The model under review builds one solid part; all positions refer to its coordinate system, in mm. A direction names the side the tool comes from. Give positions to 0.01 mm unless a question says otherwise; leave off trailing zeros. Order: outer loops, then holes, each group sorted by start corner. A loop starts at its lowest first (then second) coordinate and runs counter-clockwise, first axis right, second up. Notation, with made-up numbers: (-11, 20) - (4, 20) arc R26 ccw to (4, 56) - close; hole circle Ø1 at (55, 8). An arc over 180 degrees is marked (long way). Use CSV: the item, a comma, the result in double quotes. Start each with the question number.
1. Take a section at B-B, the plane x = 65. State the section outline as (y, z) points.
2. Machinability: for faces 1 (the flat face through (10, 13, -16)), 2 (the flat face through (61, 7, -8.5)), 3 (the flat face through (13, 8, -16)), which of the approach directions +Z, -Z, +X, -X, +Y, -Y give a long, thin tool a straight path to every point of the face, cutting with its end or side? Answer none if there is none.
3. Take a section at C-C, the plane z = -19.5. State the section outline as (x, y) points, then the cut area to 3 significant figures.
4. Draft analysis for pull direction Z (two halves, no side actions). For faces 4 (the cylindrical face through (5.81, 6.55, -15.9)), 5 (the flat face through (35, 1, 0)), 6 (the flat face through (9, 7, -46.5)), state which applies: released by +Z, released by -Z, zero draft, split by the parting line, or undercut.
5. Take a section at A-A, the plane z = -65. State the section outline as (x, y) points, then the cut area to 3 significant figures.
6. Take a section at D-D, the plane y = 6.5. State the section outline as (x, z) points.
7. For pin 1 (1 mm diameter, centred on x = 35.5, z = -20.5, fed in from -Y); pin 2 (5 mm diameter, centred on y = 7.5, z = -17, fed in from +X); pin 3 (12 mm diameter, centred on x = 55.5, z = -31.5, fed in from +Y); pin 4 (3 mm diameter, centred on x = 5.5, y = 8, fed in from +Z), all flat-tipped, find the tip position at first contact; note any pin that passes through.
8. To check wall thickness, follow line 1 (X direction, y = 2.1, z = -65); line 2 (Z direction, x = 4, y = 4.25); line 3 (Z direction, x = 65, y = 1). State the ranges of each line that lie inside material, in increasing order. Write a range as [from, to].
```python
from build123d import *

# Parameters (mm, degrees)
SKETCH1_W           = 70
SKETCH1_H           = 70
SKETCH1_R           = 1.7
PLATE_DEPTH         = 3
SKETCH2_W           = 5
SKETCH2_H           = 15
BOSS_EXTRUDE1_DEPTH = 10
FILLET1_R           = 10


with BuildPart() as part:
    # Sketch1 → Plate (new body)
    with BuildSketch(Plane(origin=(0, 0, 0), x_dir=(1, 0, 0), z_dir=(0, 1, 0))):
        with Locations((35, 35)):
            Rectangle(SKETCH1_W, SKETCH1_H)
        with Locations(Location((65, 65, 0), (0, 0, 270))):
            Circle(SKETCH1_R, mode=Mode.SUBTRACT)
        with Locations(Location((5, 65, 0), (0, 0, 90))):
            Circle(SKETCH1_R, mode=Mode.SUBTRACT)
        with Locations(Location((65, 5, 0), (0, 0, 90))):
            Circle(SKETCH1_R, mode=Mode.SUBTRACT)
        with Locations(Location((5, 5, 0), (0, 0, 270))):
            Circle(SKETCH1_R, mode=Mode.SUBTRACT)
    extrude(amount=PLATE_DEPTH)

    # Sketch2 → Boss-Extrude1 (add)
    with BuildSketch(Plane(origin=(0, 3, 0), x_dir=(1, 0, 0), z_dir=(0, 1, 0))):
        with Locations((10.5, 54)):
            Rectangle(SKETCH2_W, SKETCH2_H)
        with Locations((59.5, 54)):
            Rectangle(SKETCH2_W, SKETCH2_H)
        with Locations((10.5, 16)):
            Rectangle(SKETCH2_W, SKETCH2_H)
        with Locations((59.5, 16)):
            Rectangle(SKETCH2_W, SKETCH2_H)
    extrude(amount=BOSS_EXTRUDE1_DEPTH)

    # Fillet1
    # the kernel refuses this fillet: 10 mm, written as the material it adds along each edge
    with BuildSketch(Plane(origin=(8, 3, -22.005102572), x_dir=(-1, 0, 0), z_dir=(0, 0, -1))) as fillet1_piece_1_section:
        with BuildLine():
            CenterArc((10, 9.797958971), FILLET1_R, 180, 78.463040967)
            Line((0, 9.797958971), (-0.2, 9.797958971))
            Line((-0.2, 9.797958971), (-0.2, 0))
            Line((-0.2, 0), (0, -0.2))
            ThreePointArc((0, -0.2), (4, -0.2), (7.96, -0.195959179))
            Line((7.96, -0.195959179), (8, 0))
        make_face()
    fillet1_piece_1 = extrude(amount=39.494897428, mode=Mode.PRIVATE)
    fillet1_piece_1 = split(fillet1_piece_1, bisect_by=Plane(origin=(6.00439902, 5.286170926, -23.5), z_dir=(0, 0, 1)), keep=Keep.TOP, mode=Mode.PRIVATE)
    add(fillet1_piece_1)
    with BuildSketch(Plane(origin=(8, 3, -46.5), x_dir=(-1, 0, 0), z_dir=(0, 0, -1)), Plane(origin=(62, 3, -61.5), x_dir=(1, 0, 0), z_dir=(0, 0, 1)), Plane(origin=(8, 3, -8.5), x_dir=(-1, 0, 0), z_dir=(0, 0, -1)), Plane(origin=(62, 3, -23.5), x_dir=(1, 0, 0), z_dir=(0, 0, 1))) as fillet1_piece_2:
        with BuildLine():
            CenterArc((10, 9.797958971), FILLET1_R, 180, 78.463040967)
            Line((0, 9.797958971), (-0.2, 9.797958971))
            Line((-0.2, 9.797958971), (-0.2, 0))
            Line((-0.2, 0), (0, -0.2))
            ThreePointArc((0, -0.2), (4, -0.2), (7.96, -0.195959179))
            Line((7.96, -0.195959179), (8, 0))
        make_face()
    extrude(amount=15)
    with BuildSketch(Plane(origin=(62, 3, -61.5), x_dir=(1, 0, 0), z_dir=(0, 0, 1))) as fillet1_piece_3_section:
        with BuildLine():
            CenterArc((10, 9.797958971), FILLET1_R, 180, 78.463040967)
            Line((0, 9.797958971), (-0.2, 9.797958971))
            Line((-0.2, 9.797958971), (-0.2, 0))
            Line((-0.2, 0), (0, -0.2))
            ThreePointArc((0, -0.2), (4, -0.2), (7.96, -0.195959179))
            Line((7.96, -0.195959179), (8, 0))
        make_face()
    fillet1_piece_3 = extrude(amount=39.494897428, mode=Mode.PRIVATE)
    fillet1_piece_3 = split(fillet1_piece_3, bisect_by=Plane(origin=(63.99560098, 5.286170926, -23.5), z_dir=(0, 0, 1)), keep=Keep.TOP, mode=Mode.PRIVATE)
    add(fillet1_piece_3)
    with BuildSketch(Plane(origin=(8, 3, -8.5), x_dir=(-1, 0, 0), z_dir=(0, 0, -1))) as fillet1_piece_4_section:
        with BuildLine():
            CenterArc((10, 9.797958971), FILLET1_R, 180, 78.463040967)
            Line((0, 9.797958971), (-0.2, 9.797958971))
            Line((-0.2, 9.797958971), (-0.2, 0))
            Line((-0.2, 0), (0, -0.2))
            ThreePointArc((0, -0.2), (4, -0.2), (7.96, -0.195959179))
            Line((7.96, -0.195959179), (8, 0))
        make_face()
    fillet1_piece_4 = extrude(amount=39.494897428, mode=Mode.PRIVATE)
    fillet1_piece_4 = split(fillet1_piece_4, bisect_by=Plane(origin=(6.00439902, 5.286170926, -46.5), z_dir=(0, 0, -1)), keep=Keep.TOP, mode=Mode.PRIVATE)
    add(fillet1_piece_4)
    with BuildSketch(Plane(origin=(62, 3, -47.994897428), x_dir=(1, 0, 0), z_dir=(0, 0, 1))) as fillet1_piece_5_section:
        with BuildLine():
            CenterArc((10, 9.797958971), FILLET1_R, 180, 78.463040967)
            Line((0, 9.797958971), (-0.2, 9.797958971))
            Line((-0.2, 9.797958971), (-0.2, 0))
            Line((-0.2, 0), (0, -0.2))
            ThreePointArc((0, -0.2), (4, -0.2), (7.96, -0.195959179))
            Line((7.96, -0.195959179), (8, 0))
        make_face()
    fillet1_piece_5 = extrude(amount=39.494897428, mode=Mode.PRIVATE)
    fillet1_piece_5 = split(fillet1_piece_5, bisect_by=Plane(origin=(63.99560098, 5.286170926, -46.5), z_dir=(0, 0, -1)), keep=Keep.TOP, mode=Mode.PRIVATE)
    add(fillet1_piece_5)


solid = part.part
```
Determined:
1,outline,"(0, -70) - (3, -70) - (3, -66.7) - (0, -66.7) - close; (0, -63.3) - (3, -63.3) - (3, -61.5) - (5.66, -61.5) - (5.66, -46.5) - (3, -46.5) - (3, -23.5) - (5.66, -23.5) - (5.66, -8.5) - (3, -8.5) - (3, -6.7) - (0, -6.7) - close; (0, -3.3) - (3, -3.3) - (3, 0) - (0, 0) - close"
2,face 1,"+Z, -Z, +X, -X, +Y"
2,face 2,"+Z, +X, -X, +Y"
2,face 3,"+Z, -Z, +Y"
3,outline,"(0, 0) - (70, 0) - (70, 3) arc R10 cw to (62, 12.8) - (62, 13) - (57, 13) - (57, 3) - (13, 3) - (13, 13) - (8, 13) - (8, 12.8) arc R10 cw to (0, 3) - close"
3,area,"349 mm²"
4,face 4,"zero draft"
4,face 5,"released by +Z"
4,face 6,"undercut"
5,outline,"(0, 0) - (3.3, 0) - (3.3, 3) - (0, 3) - close; (6.7, 0) - (63.3, 0) - (63.3, 3) - (6.7, 3) - close; (66.7, 0) - (70, 0) - (70, 3) - (66.7, 3) - close"
5,area,"190 mm²"
6,outline,"(5.77, -61.5) - (13, -61.5) - (13, -46.5) - (5.77, -46.5) - close; (5.77, -23.5) - (13, -23.5) - (13, -8.5) - (5.77, -8.5) - close; (57, -61.5) - (64.23, -61.5) - (64.23, -46.5) - (57, -46.5) - close; (57, -23.5) - (64.23, -23.5) - (64.23, -8.5) - (57, -8.5) - close"
7,pin 1,"stops at y = 0"
7,pin 2,"stops at x = 65.74"
7,pin 3,"stops at y = 3"
7,pin 4,"stops at z = -8.5"
8,line 1,"x = [0, 3.3], [6.7, 63.3], [66.7, 70]"
8,line 2,"z = [-61.5, -46.5], [-23.5, -8.5]"
8,line 3,"z = [-70, -66.7], [-63.3, -6.7], [-3.3, 0]"
